For this review, use the dimensioned drawing (mm, ordinates from the lowest corner) and the shaded views. A direction names the side the tool comes from. Round coordinates to 2 decimals unless told otherwise and drop trailing zeros. Write each loop counter-clockwise with the first axis right and the second up, starting at its lowest first coordinate (ties: lowest second). Pieces come first, ordered by that corner, then holes. Notation, with made-up numbers: (23, -27) - (72, -27) arc R23 cw to (72, -7) - close; hole circle Ø3 at (87, 35). An arc over 180 degrees is marked (long way). Write each question's results on one line, items separated by ' | '.
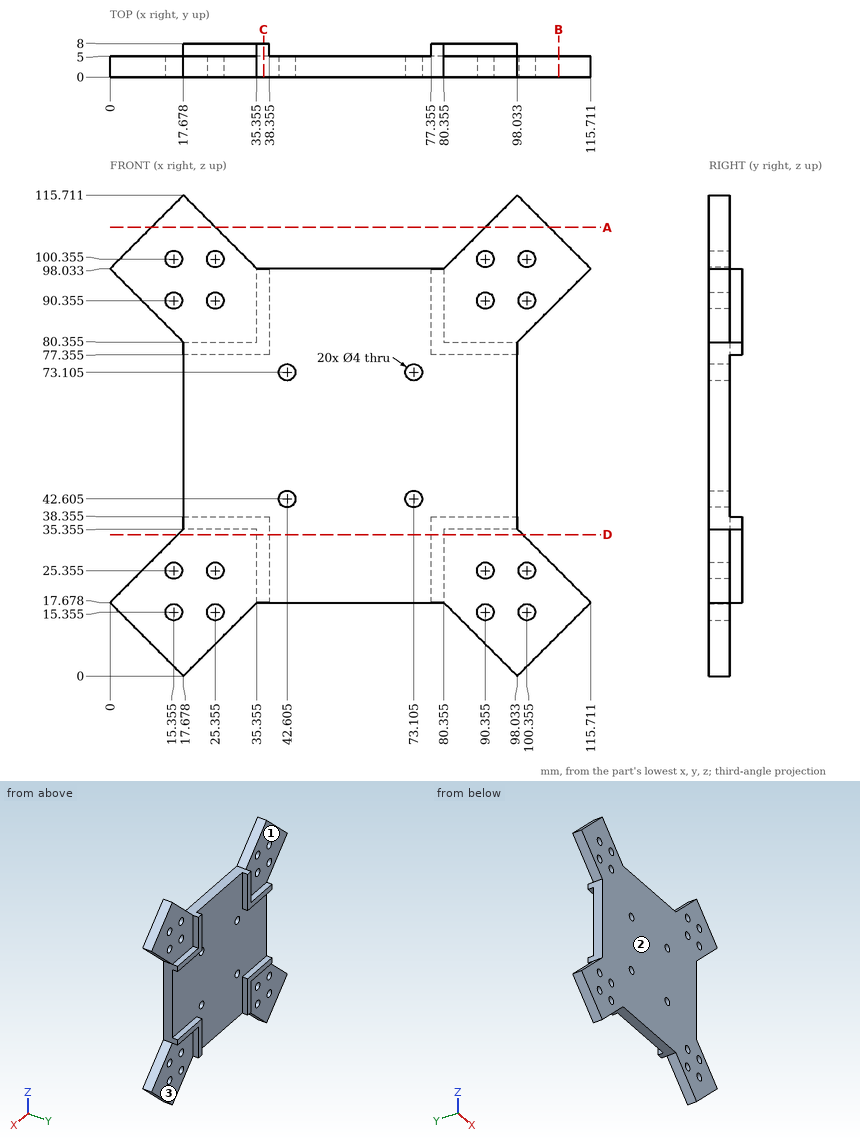
Q1. Tool access review of the marked faces 1, 2 and 3: name each direction out of +Z, -Z, +X, -X, +Y, -Y from which nothing blocks a thin tool from reaching the whole face with its end or side.
Evaluation:
face 1: +Z, -X, +Y | face 2: +Z, -Z, +X, -X, -Y | face 3: -Z, +X, +Y
Q2. We need section B-B (x = 108). State the section outline as (y, z) points, plus the area to 3 significant figures.
Evaluation:
outline: (0, 9.97) - (5, 9.97) - (5, 25.39) - (0, 25.39) - close; (0, 90.32) - (5, 90.32) - (5, 105.74) - (0, 105.74) - close | area: 154 mm^2
Q3. We need section D-D (z = 34). State the section outline as (x, y) points (1 decimal).
Evaluation:
outline: (16.3, 0) - (99.4, 0) - (99.4, 5) - (80.4, 5) - (80.4, 8) - (77.4, 8) - (77.4, 5) - (38.4, 5) - (38.4, 8) - (35.4, 8) - (35.4, 5) - (16.3, 5) - close
Q4. We need section A-A (z = 108). State the section outline as (x, y) points, plus the area to 3 significant figures.
Evaluation:
outline: (9.97, 0) - (25.39, 0) - (25.39, 5) - (9.97, 5) - close; (90.32, 0) - (105.74, 0) - (105.74, 5) - (90.32, 5) - close | area: 154 mm^2
Q5. For probe 1 along Z at (x, y) = (73, 2); probe 2 along X at (y, z) = (4.25, 99) (1 decimal); probe 3 along X at (y, z) = (6, 24.5) (1 decimal), list the stretches that pass through material, from the lowest coordinate up.
Evaluation:
probe 1: z = 17.68 to 40.61, 44.6 to 71.11, 75.1 to 98.03 | probe 2: x = 1 to 13.9, 16.8 to 23.9, 26.8 to 34.4, 81.3 to 88.9, 91.8 to 98.9, 101.8 to 114.7 | probe 3: x = 35.4 to 38.4, 77.4 to 80.4
Q6. Insertion check: P1, Ø3.5, axis at y = 7, z = 28.5, coming from the +X side (1 decimal); P2, Ø1.5, axis at x = 45.5, y = 2.5, coming from the +Z side; P3, Ø12, axis at x = 56.5, z = 45, coming from the +Y side; P4, Ø3, axis at x = 90.36, z = 100.36, coming from the -Y side. Each pin has a flat end and moves straight along its axis. Give the tip position at first contact, or say it passes through.
Evaluation:
P1: stops at x = 80.4 | P2: stops at z = 98.03 | P3: stops at y = 5 | P4: passes through
Q7. We need section C-C (x = 37). State the section outline as (y, z) points (1 decimal), plus the area to 3 significant figures.
Evaluation:
outline: (0, 17.7) - (8, 17.7) - (8, 38.4) - (5, 38.4) - (5, 77.4) - (8, 77.4) - (8, 98) - (0, 98) - close | area: 526 mm^2
